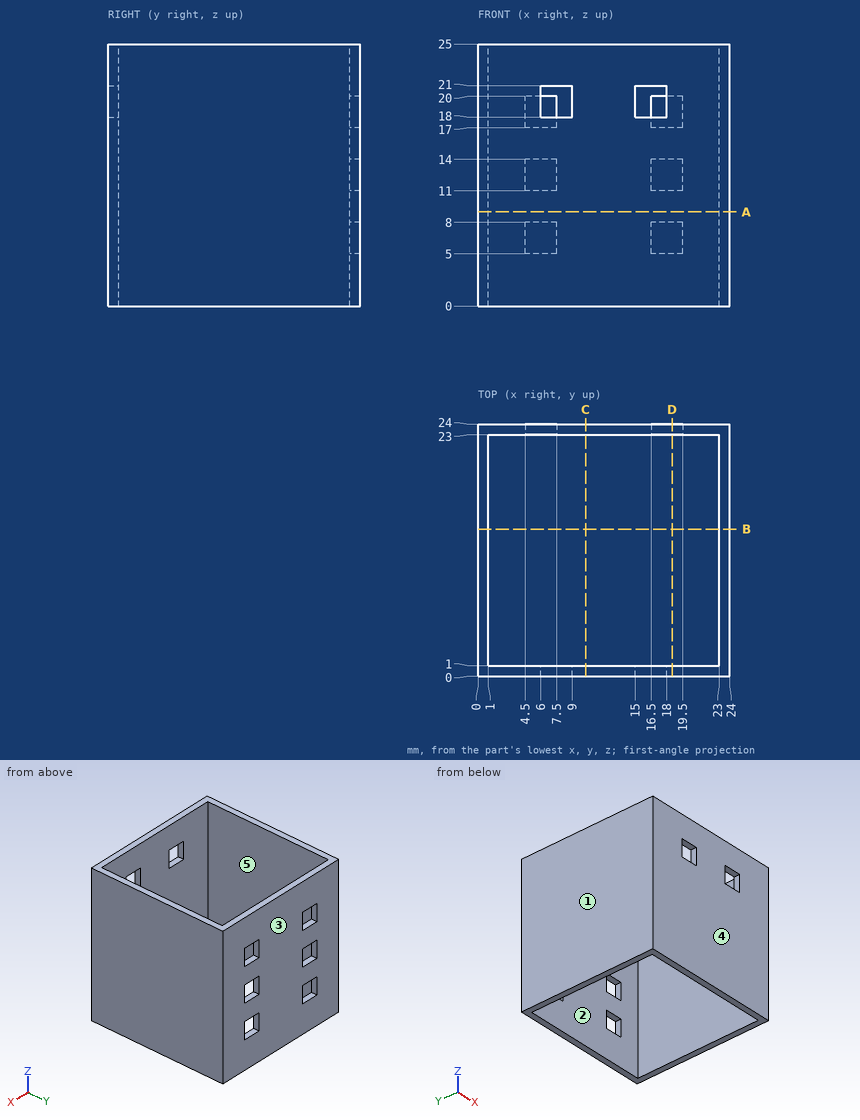
Verification items for this drawing (mm, ordinates from the low corner). A direction names the side the tool comes from. Give positions to 0.01 mm unless a question says otherwise; leave off trailing zeros. Write each loop counter-clockwise with the first axis right and the second up, starting at its lowest first coordinate (ties: lowest second). Pieces come first, ordered by that corner, then holes. Notation, with made-up numbers: (86.25, 53.25) -> (106.25, 53.25) arc R4 ccw to (106.25, 57.25) -> close; hole circle Ø5 at (86, 10.25). An arc over 180 degrees is marked (long way). Use CSV: the item, a comma, the result in double quotes. Start each with the question number.
Q1. Scan line: line 1 along Y through (x, z) = (11.5, 15.5). Record every from-to range of solid material in increasing order.
Q2. Release check for a two-part mould opening along Y. For the marked faces 3, 4 and 5 record: +Y half, -Y half, draft (parallel to the pull), parting line (faces both ways), or undercut.
Q3. Cross-section at D-D on x = 18.5. Enter the section's corners in (y, z), and give its area (3 significant figures).
Q4. Cross-section at A-A on z = 9. Enter the section's corners in (x, y).
Q5. Tool access check on the marked faces 1 and 2. Record the directions out of +Z, -Z, +X, -X, +Y, -Y that give a thin tool (end or side, any length) a straight path to the whole face; none if there is none.
Q6. Cross-section at B-B on y = 14. Enter the section's corners in (x, z).
Working result:
1,line 1,"y = 0 to 1, 23 to 24"
2,face 3,"+Y half"
2,face 4,"-Y half"
2,face 5,"undercut"
3,outline,"(0, 0) -> (1, 0) -> (1, 25) -> (0, 25) -> close; (23, 0) -> (24, 0) -> (24, 5) -> (23, 5) -> close; (23, 8) -> (24, 8) -> (24, 11) -> (23, 11) -> close; (23, 14) -> (24, 14) -> (24, 17) -> (23, 17) -> close; (23, 20) -> (24, 20) -> (24, 25) -> (23, 25) -> close"
3,area,"41.0 mm^2"
4,outline,"(0, 0) -> (24, 0) -> (24, 24) -> (0, 24) -> close; hole (1, 1) -> (23, 1) -> (23, 23) -> (1, 23) -> close"
5,face 1,"+Z, -Z, -X, +Y, -Y"
5,face 2,"+Z, -Z"
6,outline,"(0, 0) -> (1, 0) -> (1, 25) -> (0, 25) -> close; (23, 0) -> (24, 0) -> (24, 25) -> (23, 25) -> close"
